Autodesk Inventor part; units mm, degrees
ref_plane "YZ Plane" through (0, 0, 0) normal (1, 0, 0) x (0, 1, 0)
ref_plane "XZ Plane" through (0, 0, 0) normal (0, 1, 0) x (-1, 0, 0)
ref_plane "XY Plane" through (0, 0, 0) normal (0, 0, 1) x (1, 0, 0)
sketch "Sketch2" plane through (0, 0, 0) normal (0, 0, 1) x (1, 0, 0)
  point P0 (0, 0)
  point P1 (-17.5, 0)
  dimension "d6" = 17.5
sketch "Sketch1" plane through (0, 0, 0) normal (0, 0, 1) x (1, 0, 0)
  arc A0 (-17.5, -4.899) -> (-17.5, 4.899) centre (-22.5, 0) ccw
  arc A1 (-17.5, 4.899) -> (-17.5, -4.899) centre (-12.5, 0) ccw
  line L0 (-15.5, 0) -> (-15.5, 11.1541) construction
  point P0 (-17.5, 0)
  dimension "d3" = 14
  dimension "d4" = 14
  dimension "d5" = 10
  dimension "d7" = 2
extrude "Extrusion1" add sketch "Sketch1" along normal blind 1
sketch "Sketch3" plane through (0, 0, 1) normal (0, 0, 1) x (1, 0, 0)
  point P0 (0, 0)
  point P1 (-17.5, 0)
  point P2 (-17.5, 2)
  point P3 (-17.5, -2)
  dimension "d10" = 2
  dimension "d11" = 2
hole "Hole1" at (-17.5, 2, 1) at (-17.5, -2, 1) direction (0, 0, -1) diameter 1.5 end through all
fillet "Fillet1" radius 0.5 2 edges at (-17.5, -4.899, 0.5) (-17.5, 4.899, 0.5)
properties part number "phalanx 3 spring pins support"
Can you work these out from the model? Positions are in its coordinate system, mm. Round coordinates to 2 decimals unless told otherwise and drop trailing zeros. Order: outer loops, then holes, each group sorted by start corner. A loop starts at its lowest first (then second) coordinate and runs counter-clockwise, first axis right, second up. Notation, with made-up numbers: M 70,70.25 L 118,70.25 A16 cw 118,83.25 Z; hole C -38,-36.75 d6. An arc over 180 degrees is marked long. Use a Markdown table: item, result.
1) If I drill on line 1 along Y through (x, z) = (-17.5, 0.4); line 2 along Y through (x, z) = (-17, 0.7); line 3 along X through (y, z) = (-1.5, 0.8), over which ranges is the centre line in solid material (lowest first)?
Geometry says:
| item | result |
|---|---|
| line 1 | y = -4.65 to -2.75, -1.25 to 1.25, 2.75 to 4.65 |
| line 2 | y = -4.33 to -2.56, -1.44 to 1.44, 2.56 to 4.33 |
| line 3 | x = -19.34 to -18.06, -16.94 to -15.66 |
2) Imagine slicing it at B-B (y = -2). List the corners of the cut face in (x, z) for me.
Geometry says:
| item | result |
|---|---|
| outline | M -19.21,0 L -18.25,0 L -18.25,1 L -19.21,1 Z; M -16.75,0 L -15.79,0 L -15.79,1 L -16.75,1 Z |
3) I'm going to push a flat-ended pin straight in: P1, Ø1.2, axis at x = -17.5, y = -2, coming from the -Z side. Where does the tip first touch, or does it pass through?
Geometry says:
| item | result |
|---|---|
| P1 | passes through |
4) Imagine slicing it at C-C (z = 0.2). Give the number of separate pieces and of enclosed holes in the cut face, then the cut area to 3 significant figures.
Geometry says:
| item | result |
|---|---|
| separate pieces | 1 |
| enclosed holes | 2 |
| area | 23.3 mm² |
5) Imagine slicing it at A-A (x = -18.15). List the corners of the cut face in (y, z) for me.
Geometry says:
| item | result |
|---|---|
| outline | M -4.13,0 L -2.37,0 L -2.37,1 L -4.13,1 Z; M -1.63,0 L 1.63,0 L 1.63,1 L -1.63,1 Z; M 2.37,0 L 4.13,0 L 4.13,1 L 2.37,1 Z |
6) If we mould it in two halves opening along X, with no side actions, what happens to faces 1 (the face through (-18, 0, 0)), 2 (the face through (-15.5, 0.1, 0.5)), 3 (the face through (-16.768, 2.163, 0.493))? For each: +X half, -X half, draft (parallel to the pull), parting line (faces both ways), or undercut.
Geometry says:
| item | result |
|---|---|
| face 1 | draft |
| face 2 | +X half |
| face 3 | undercut |
